Could you check a few things on this model? Use its own coordinates, in mm. Face numbers are marked on the shaded views. A direction names the side the tool comes from. Give positions to 0.01 mm unless a question says otherwise; leave off trailing zeros. Order: outer loops, then holes, each group sorted by start corner. A loop starts at its lowest first (then second) coordinate and runs counter-clockwise, first axis right, second up. Notation, with made-up numbers: (11.5, 43) - (15.5, 43) arc R16 ccw to (15.5, 49) - close; hole circle Ø9 at (5, 75.25). An arc over 180 degrees is marked (long way). Put each result on its own line as item: value.
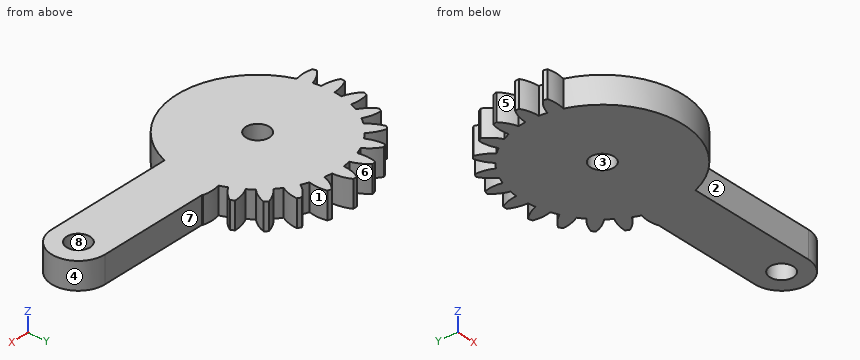
from build123d import *

# Parameters (mm, degrees)
SKETCH1_R           = 1.75
BOSS_EXTRUDE1_DEPTH = 4


with BuildPart() as part:
    # Sketch1 → Boss-Extrude1 (new body)
    with BuildSketch(Plane.XY):
        with BuildLine():
            ThreePointArc((30.75, -4), (34.75, 0), (30.75, 4))
            Line((30.75, 4), (14.072558403, 4))
            ThreePointArc((14.072558403, 4), (14.06038767, 4.04257326), (14.048088143, 4.085109489))
            ThreePointArc((14.048088143, 4.085109489), (12.712915648, 4.255390909), (11.377106712, 4.090176385))
            ThreePointArc((11.377106712, 4.090176385), (11.169703548, 4.626642697), (10.937020765, 5.152637848))
            ThreePointArc((10.937020765, 5.152637848), (11.998404632, 5.980373095), (12.82210701, 7.044889767))
            ThreePointArc((12.82210701, 7.044889767), (12.669951657, 7.315), (12.51210701, 7.581825517))
            ThreePointArc((12.51210701, 7.581825517), (11.17835734, 7.400736668), (9.930825655, 6.8954189))
            ThreePointArc((9.930825655, 6.8954189), (9.591641884, 7.359925677), (9.230750012, 7.807775241))
            ThreePointArc((9.230750012, 7.807775241), (10.041734454, 8.882012453), (10.561852666, 10.123446462))
            ThreePointArc((10.561852666, 10.123446462), (10.344972209, 10.344972209), (10.123446462, 10.561852666))
            ThreePointArc((10.123446462, 10.561852666), (8.882012453, 10.041734454), (7.807775241, 9.230750012))
            ThreePointArc((7.807775241, 9.230750012), (7.359925677, 9.591641884), (6.8954189, 9.930825655))
            ThreePointArc((6.8954189, 9.930825655), (7.400736668, 11.17835734), (7.581825517, 12.51210701))
            ThreePointArc((7.581825517, 12.51210701), (7.315, 12.669951657), (7.044889767, 12.82210701))
            ThreePointArc((7.044889767, 12.82210701), (5.980373095, 11.998404632), (5.152637848, 10.937020765))
            ThreePointArc((5.152637848, 10.937020765), (4.626642697, 11.169703548), (4.090176385, 11.377106712))
            ThreePointArc((4.090176385, 11.377106712), (4.255390909, 12.712915648), (4.085109489, 14.048088143))
            ThreePointArc((4.085109489, 14.048088143), (3.78652263, 14.131494839), (3.486235477, 14.208555951))
            ThreePointArc((3.486235477, 14.208555951), (2.671181194, 13.137403362), (2.1463567, 11.897951627))
            ThreePointArc((2.1463567, 11.897951627), (1.578061664, 11.986568374), (1.00619511, 12.048056748))
            ThreePointArc((1.00619511, 12.048056748), (0.820047291, 13.381109763), (0.31, 14.626715284))
            ThreePointArc((0.31, 14.626715284), (0, 14.63), (-0.31, 14.626715284))
            ThreePointArc((-0.31, 14.626715284), (-0.820047291, 13.381109763), (-1.00619511, 12.048056748))
            ThreePointArc((-1.00619511, 12.048056748), (-1.578061664, 11.986568374), (-2.1463567, 11.897951627))
            ThreePointArc((-2.1463567, 11.897951627), (-2.671181194, 13.137403362), (-3.486235477, 14.208555951))
            ThreePointArc((-3.486235477, 14.208555951), (-3.78652263, 14.131494839), (-4.085109489, 14.048088143))
            ThreePointArc((-4.085109489, 14.048088143), (-4.255390909, 12.712915648), (-4.090176385, 11.377106712))
            ThreePointArc((-4.090176385, 11.377106712), (-4.626642697, 11.169703548), (-5.152637848, 10.937020765))
            ThreePointArc((-5.152637848, 10.937020765), (-5.980373095, 11.998404632), (-7.044889767, 12.82210701))
            ThreePointArc((-7.044889767, 12.82210701), (-7.315, 12.669951657), (-7.581825517, 12.51210701))
            ThreePointArc((-7.581825517, 12.51210701), (-7.400736668, 11.17835734), (-6.8954189, 9.930825655))
            ThreePointArc((-6.8954189, 9.930825655), (-7.359925677, 9.591641884), (-7.807775241, 9.230750012))
            ThreePointArc((-7.807775241, 9.230750012), (-8.882012453, 10.041734454), (-10.123446462, 10.561852666))
            ThreePointArc((-10.123446462, 10.561852666), (-10.344972209, 10.344972209), (-10.561852666, 10.123446462))
            ThreePointArc((-10.561852666, 10.123446462), (-10.041734454, 8.882012453), (-9.230750012, 7.807775241))
            ThreePointArc((-9.230750012, 7.807775241), (-9.591641884, 7.359925677), (-9.930825655, 6.8954189))
            ThreePointArc((-9.930825655, 6.8954189), (-11.17835734, 7.400736668), (-12.51210701, 7.581825517))
            ThreePointArc((-12.51210701, 7.581825517), (-12.669951657, 7.315), (-12.82210701, 7.044889767))
            ThreePointArc((-12.82210701, 7.044889767), (-11.998404632, 5.980373095), (-10.937020765, 5.152637848))
            ThreePointArc((-10.937020765, 5.152637848), (-11.169703548, 4.626642697), (-11.377106712, 4.090176385))
            ThreePointArc((-11.377106712, 4.090176385), (-12.712915648, 4.255390909), (-14.048088143, 4.085109489))
            ThreePointArc((-14.048088143, 4.085109489), (-14.131494839, 3.78652263), (-14.208555951, 3.486235477))
            ThreePointArc((-14.208555951, 3.486235477), (-13.137403362, 2.671181194), (-11.897951627, 2.1463567))
            ThreePointArc((-11.897951627, 2.1463567), (-11.986568374, 1.578061664), (-12.048056748, 1.00619511))
            ThreePointArc((-12.048056748, 1.00619511), (-13.381109763, 0.820047291), (-14.626715284, 0.31))
            ThreePointArc((-14.626715284, 0.31), (-14.63, 0), (-14.626715284, -0.31))
            ThreePointArc((-14.626715284, -0.31), (-13.381109763, -0.820047291), (-12.048056748, -1.00619511))
            ThreePointArc((-12.048056748, -1.00619511), (-11.986568374, -1.578061664), (-11.897951627, -2.1463567))
            ThreePointArc((-11.897951627, -2.1463567), (-13.137403362, -2.671181194), (-14.208555951, -3.486235477))
            ThreePointArc((-14.208555951, -3.486235477), (-14.131494839, -3.78652263), (-14.048088143, -4.085109489))
            ThreePointArc((-14.048088143, -4.085109489), (-12.712915648, -4.255390909), (-11.377106712, -4.090176385))
            ThreePointArc((-11.377106712, -4.090176385), (0.047845736, -12.089905326), (11.409123542, -4))
            Line((11.409123542, -4), (30.75, -4))
        make_face()
        Circle(SKETCH1_R, mode=Mode.SUBTRACT)
        with Locations((30.75, 0)):
            Circle(SKETCH1_R, mode=Mode.SUBTRACT)
    extrude(amount=BOSS_EXTRUDE1_DEPTH)


solid = part.part
1) Suppose I cut it at A-A, the plane z = 2.2. State how many separate pieces and enclosed holes the cut face has, and give its area (3 significant figures).
Filled in:
separate pieces: 1
enclosed holes: 2
area: 664 mm^2
2) If I drill on line 1 (Y direction, x = 30.75, z = 1.2); line 2 (X direction, y = 11.5, z = 0.9); line 3 (Y direction, x = 0, z = 1.8), over which ranges is the centre line in solid material (lowest first)? Write a range as [from, to].
Filled in:
line 1: y = [-4, -1.75], [1.75, 4]
line 2: x = [-7.48, -5.54], [-4.12, 4.12], [5.54, 7.48]
line 3: y = [-12.09, -1.75], [1.75, 14.63]
3) We'd pull the mould along Y, two halves only. Please class the marked faces 1, 2, 3 and 4: pulls with the +Y half, pulls with the -Y half, needs draft (parallel to the pull), parting line crosses it, or undercut.
Filled in:
face 1: undercut
face 2: pulls with the -Y half
face 3: undercut
face 4: parting line crosses it
4) Suppose I cut it at B-B, the plane y = -6.75. List the corners of the cut face in (x, z) for me, and give its area (3 significant figures).
Filled in:
outline: (-10.03, 0) - (10.03, 0) - (10.03, 4) - (-10.03, 4) - close
area: 80.2 mm^2
5) Suppose I cut it at C-C, the plane y = 6. List the corners of the cut face in (x, z) for me, and give its area (3 significant figures).
Filled in:
outline: (-12.02, 0) - (12.02, 0) - (12.02, 4) - (-12.02, 4) - close
area: 96.1 mm^2
6) I'm going to push flat-ended pins straight in: pin 1 (1.5 mm diameter, centred on x = 21, z = 3, fed in from -Y); pin 2 (3 mm diameter, centred on x = 0, y = 0, fed in from +Z). Where does each tip first touch, or does it pass through?
Filled in:
pin 1: stops at y = -4
pin 2: passes through
7) Which directions (+Z, -Z, +X, -X, +Y, -Y) give clear straight access to the entire face, cutting with the end or side of a thin tool? Please do the marked faces 5, 6, 7 and 8.
Filled in:
face 5: +Z, -Z, -X
face 6: +Z, -Z, +Y
face 7: +Z, -Z, +X, +Y
face 8: +Z, -Z
